Solid Edge part; units mm, degrees
sketch "Sketch1" plane through (-4, 0, 0) normal (1, 0, 0) x (0, 1, 0)
  arc A0 (1.5681, 3.7871) -> (0.7, 3.2503) centre (1.3, 3.2503) ccw
  line L0 (0.7, 3.2503) -> (0.7, 2.8302)
  arc A1 (0.7, 2.8302) -> (0.4776, 2.5404) centre (0.4, 2.8302) cw
  line L1 (0.4776, 2.5404) -> (0.2224, 2.472)
  arc A2 (0.2224, 2.472) -> (0, 2.1822) centre (0.3, 2.1822) ccw
  line L2 (0, 2.1822) -> (0, -2.1822)
  arc A3 (0, -2.1822) -> (0.2224, -2.472) centre (0.3, -2.1822) ccw
  line L3 (0.2224, -2.472) -> (0.4776, -2.5404)
  arc A4 (0.4776, -2.5404) -> (0.7, -2.8302) centre (0.4, -2.8302) cw
  line L4 (0.7, -2.8302) -> (0.7, -3.2503)
  arc A5 (0.7, -3.2503) -> (1.5681, -3.7871) centre (1.3, -3.2503) ccw
  arc A6 (1.5681, -3.7871) -> (4.4916, -1.0434) centre (-1.5598, 2.4752) ccw
  arc A7 (4.4916, -1.0434) -> (4.6, -0.6413) centre (3.8, -0.6413) ccw
  line L5 (4.6, -0.6413) -> (4.6, 0.6413)
  arc A8 (4.6, 0.6413) -> (4.4916, 1.0434) centre (3.8, 0.6413) ccw
  arc A9 (4.4916, 1.0434) -> (1.5681, 3.7871) centre (-1.5598, -2.4752) ccw
extrude "ExtrudedProtrusion_1" add sketch "Sketch1" along normal blind 12
sketch "Sketch2" plane through (0, 0, 0) normal (1, 0, 0) x (0, 1, 0)
  line L0 (0, 0) -> (0, 2.5)
  line L1 (0, 2.5) -> (0.433, 2.067)
  line L2 (0.433, 2.067) -> (4.167, 2.067)
  line L3 (4.167, 2.067) -> (4.6, 2.5)
  line L4 (4.6, 2.5) -> (4.6, 0)
  line L5 (4.6, 0) -> (0, 0)
revolve "RevolvedCutout1" cut sketch "Sketch2" angle 360 about axis through (0, 4.6, 0) along (0, -1, 0)
sketch "Sketch3" plane through (0, 0, 0) normal (0, 0, 1) x (1, 0, 0)
  arc A0 (5, 2.2) -> (5, 5.2) centre (5, 3.7) cw
  line L0 (5, 5.2) -> (5, 2.2)
revolve "RevolvedProtrusion1" add sketch "Sketch3" angle 360 about axis through (5, 5.2, 0) along (0, -1, 0)
properties part number "150914 NST-5-M5"
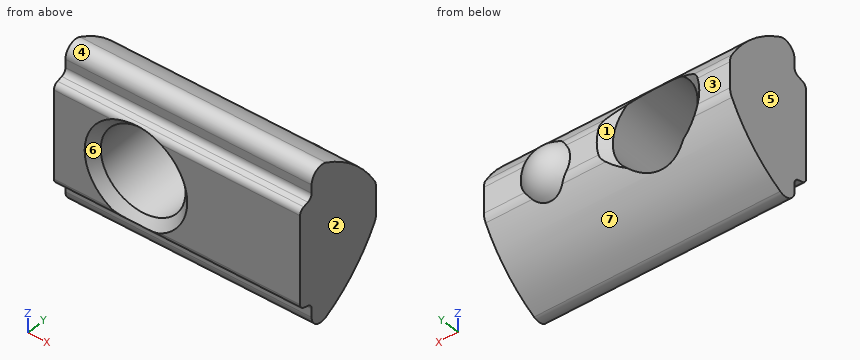
Can you work these out from the model? Positions are in its coordinate system, mm. Face numbers are marked on the shaded views. A direction names the side the tool comes from. Round coordinates to 2 decimals unless told otherwise and drop trailing zeros. Order: outer loops, then holes, each group sorted by start corner. A loop starts at its lowest first (then second) coordinate and runs counter-clockwise, first axis right, second up. Notation, with made-up numbers: (-30.5, 61.5) -> (1.5, 61.5) arc R10 ccw to (1.5, 72.5) -> close; hole circle Ø3 at (81, 18). An arc over 180 degrees is marked (long way). Return JSON: item names as keys, results as strings. Group by question number.
1. Which directions (+Z, -Z, +X, -X, +Y, -Y) give clear straight access to the entire face, cutting with the end or side of a thin tool? Please do the marked faces 1, 2 and 3.
2. Will these pins go through, and if not, where does the flat tip stop? pin 1 (1 mm diameter, centred on x = -1.5, y = 3.5, fed in from +Z); pin 2 (1 mm diameter, centred on x = -3, z = -0.5, fed in from +Y); pin 3 (1.5 mm diameter, centred on x = 6, y = 2, fed in from +Z).
3. We'd pull the mould along Z, two halves only. Please class the marked faces 4, 5, 6 and 7: released by +Z, released by -Z, zero draft, split by the parting line, or undercut.
4. I need wall thicknesses on line 1 (X direction, y = 2.9, z = 0); line 2 (Y direction, x = 2.75, z = -0.5); line 3 (Z direction, x = 1.25, y = 0.55). Which ranges of each line are inside material? Lowest first, please. Write a range as [from, to].
5. If we section it at B-B, the plane x = 0: Write out the boundary of the cut face in (y, z).
6. If we section it at A-A, the plane z = 0: Write out the boundary of the cut face in (x, y).
7. If we section it at C-C, the plane y = 3.95: Write out the boundary of the cut face in (x, z), then the cut area to 3 significant figures.
8. If we section it at D-D, the plane y = 3.25: Write out the boundary of the cut face in (x, z).
Output values:
{
 "1": {"face 1": "+Y", "face 2": "+Z, -Z, +X, +Y, -Y", "face 3": "+Z, -Z, -X, +Y"},
 "2": {"pin 1": "z = 2.84", "pin 2": "y = 4.6", "pin 3": "z = 3.85"},
 "3": {"face 4": "released by +Z", "face 5": "zero draft", "face 6": "undercut", "face 7": "released by -Z"},
 "4": {"line 1": "[-4, -2.07], [2.07, 8]", "line 2": "[0, 4.6]", "line 3": "[-2.57, -1.65], [1.65, 2.57]"},
 "5": {"outline": "(0.1, -2.4) arc R0.3 ccw to (0.22, -2.47) -> (0.48, -2.54) arc R0.3 cw to (0.7, -2.83) -> (0.7, -3.25) arc R0.6 ccw to (1.57, -3.79) arc R7 ccw to (3.77, -2.07) -> (0.43, -2.07) -> close; (0.1, 2.4) -> (0.43, 2.07) -> (3.77, 2.07) arc R7 ccw to (1.57, 3.79) arc R0.6 ccw to (0.7, 3.25) -> (0.7, 2.83) arc R0.3 cw to (0.48, 2.54) -> (0.22, 2.47) arc R0.3 ccw to start"},
 "6": {"outline": "(-4, 0) -> (-2.5, 0) -> (-2.07, 0.43) -> (-2.07, 4.17) -> (-2.5, 4.6) -> (-4, 4.6) -> close; (2.07, 0.43) -> (2.5, 0) -> (8, 0) -> (8, 4.6) -> (6.2, 4.6) arc R1.5 ccw to (3.8, 4.6) -> (2.5, 4.6) -> (2.07, 4.17) -> close"},
 "7": {"outline": "(-4, -1.84) -> (-0.94, -1.84) arc R2.07 cw to (-0.94, 1.84) -> (-4, 1.84) -> close; (0.94, -1.84) -> (8, -1.84) -> (8, 1.84) -> (0.94, 1.84) arc R2.07 cw to start", "area": "31.4 mm²"},
 "8": {"outline": "(-4, -2.61) -> (8, -2.61) -> (8, 2.61) -> (-4, 2.61) -> close; hole circle Ø4.13 at (0, 0)"}
}
